Verification items for the finished model (mm, model axes). Face numbers are marked on the shaded views. A direction names the side the tool comes from. Give positions to 0.01 mm unless a question says otherwise; leave off trailing zeros. Loops run counter-clockwise (first coordinate to the right, second up) from the corner with the lowest first, then second, coordinate; pieces in that order, holes last. Notation, with made-up numbers: (16.25, 7) - (44.25, 7) arc R19 cw to (44.25, 30) - close; hole circle Ø6 at (14, 35). An arc over 180 degrees is marked (long way). Answer in a Markdown table with one row per item.
Autodesk Inventor part; units mm, degrees
sketch "Sketch1" plane through (0, 0, 0) normal (0, 0, 1) x (1, 0, 0)
  line L0 (0, 2.5316) -> (0, -2.5316) construction
  line L1 (-5.1172, 0) -> (5.1172, 0) construction
  circle A0 centre (0, 0) radius 15.5
  dimension "d0" = 31
extrude "Extrusion1" add sketch "Sketch1" along normal blind 2
sketch "Sketch2" plane through (0, 0, 2) normal (0, 0, 1) x (1, 0, 0)
  circle A0 centre (0, 0) radius 13
  line L0 (0, 0) -> (0, 13)
  line L1 (0, 0) -> (13, 0)
  line L2 (0, 0) -> (0, -13)
  line L3 (0, 0) -> (-13, 0)
  circle A1 centre (-13, 0) radius 2.25
  circle A2 centre (0, 13) radius 2.25
  circle A3 centre (13, 0) radius 2.25
  circle A4 centre (0, -13) radius 2.25
  dimension "d3" = 26
  dimension "d4" = 4.5
  dimension "d5" = 4.5
  dimension "d6" = 4.5
  dimension "d7" = 4.5
extrude "Extrusion2" add sketch "Sketch2" along normal blind 5 contours L1 A3 A0 | A0 A3 | A0 A3 L1 | A2 L0 A0 | A0 A2 | A4 A0 | A0 L2 A4 | L0 A2 A0 | A0 A4 L2 | A1 A0 L3 | L3 A0 A1 | A0 A1
chamfer "Chamfer1" distance 1 distance2 4.5 1 edges at (-15.25, 0, 7) measured on face at (-13.6641, 0.3485, 7)
chamfer "Chamfer2" distance 1 distance2 4.5 1 edges at (-2.25, -13, 7) measured on face at (-0.0904, -12.342, 7)
chamfer "Chamfer3" distance 1 distance2 4.5 1 edges at (10.75, 0, 7) measured on face at (12.3359, 0.3485, 7)
chamfer "Chamfer4" distance 1 distance2 4.5 1 edges at (-2.25, 13, 7) measured on face at (-0.0904, 13.658, 7)
properties part number "Kogel houder2" material "S235"
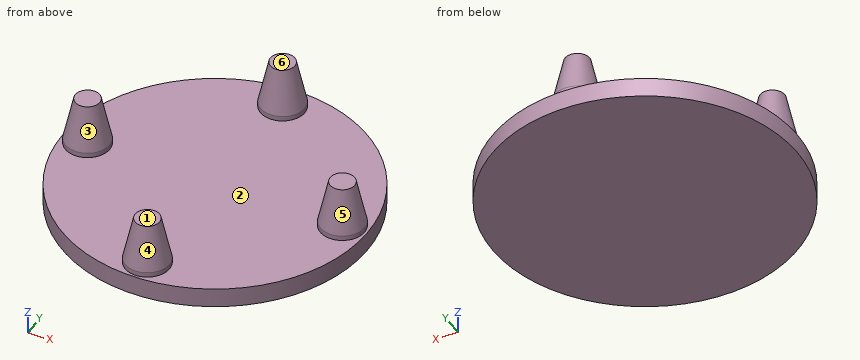
Q1. Sectioned sample at B-B (z = 4.75). Record the cut outline in (x, y).
Completed:
| item | result |
|---|---|
| outline | circle Ø3.5 at (-13, 0); circle Ø3.5 at (0, -13); circle Ø3.5 at (0, 13); circle Ø3.5 at (13, 0) |
Q2. Go/stop test with flat-tipped pins: P1, Ø15.5, axis at x = 5, y = -1.5, coming from the +Z side; P2, Ø1, axis at x = 1, z = 5, coming from the -Y side; P3, Ø3, axis at x = -12, z = 5, coming from the +Y side. Record where each tip stops, or that it passes through.
Completed:
| item | result |
|---|---|
| P1 | z = 7 |
| P2 | y = -14.66 |
| P3 | y = 1.97 |
Q3. Tool access check on the marked faces 1 and 2. Record the directions out of +Z, -Z, +X, -X, +Y, -Y that give a thin tool (end or side, any length) a straight path to the whole face; none if there is none.
Completed:
| item | result |
|---|---|
| face 1 | +Z, +X, -X, +Y, -Y |
| face 2 | +Z |
Q4. Sectioned sample at D-D (z = 0.5). Record the cut outline in (x, y), and give its area (3 significant figures).
Completed:
| item | result |
|---|---|
| outline | circle Ø31 at (0, 0) |
| area | 755 mm^2 |
Q5. Thickness scan on line 1 (Z direction, x = -10, y = 2.5); line 2 (X direction, y = 0.5, z = 3); line 3 (Y direction, x = 0.5, z = 1.75). Record the ranges inside material, lowest first.
Completed:
| item | result |
|---|---|
| line 1 | 0 to 2 |
| line 2 | -15.08 to -10.92, 10.92 to 15.08 |
| line 3 | -15.49 to 15.49 |
Q6. Sectioned sample at A-A (y = 0). Record the cut outline in (x, z).
Completed:
| item | result |
|---|---|
| outline | (-15.5, 0) - (15.5, 0) - (15.5, 2) - (15.25, 2) - (15.25, 2.5) - (14.25, 7) - (11.75, 7) - (10.75, 2.5) - (10.75, 2) - (-10.75, 2) - (-10.75, 2.5) - (-11.75, 7) - (-14.25, 7) - (-15.25, 2.5) - (-15.25, 2) - (-15.5, 2) - close |
Q7. Draft check along X on the marked faces 3, 4, 5 and 6. Enter one of: +X half, -X half, draft (parallel to the pull), parting line (faces both ways), or undercut.
Completed:
| item | result |
|---|---|
| face 3 | undercut |
| face 4 | parting line |
| face 5 | undercut |
| face 6 | draft |
